Autodesk Fusion 360 part; units mm, degrees
sketch "Skizze1" plane through (0, 0, 0) normal (0, 1, 0) x (1, 0, 0)
  line L0 (7, -7) -> (-7, -7)
  line L1 (-7, -7) -> (-7, 7)
  line L2 (-7, 7) -> (7, 7)
  line L3 (7, 7) -> (7, -7)
  line L4 (7, -7) -> (-7, 7) construction
  line L5 (-7, -7) -> (7, 7) construction
  line L6 (6, 1.65) -> (7, 1.65)
  line L7 (7, 1.65) -> (7, -1.65)
  line L8 (7, -1.65) -> (6, -1.65)
  line L9 (6, -1.65) -> (6, 1.65)
  line L10 (0, 0) -> (-0.0828, 0.0828)
  line L11 (0, 0) -> (0, 4.3114) construction
  line L12 (-7, -1.65) -> (-6, -1.65)
  line L13 (-6, -1.65) -> (-6, 1.65)
  line L14 (-7, 1.65) -> (-7, -1.65)
  line L15 (-6, 1.65) -> (-7, 1.65)
  line L16 (8, -8) -> (-8, -8) construction
  line L17 (-8, -8) -> (-8, 8) construction
  line L18 (-8, 8) -> (8, 8) construction
  line L19 (8, 8) -> (8, -8) construction
  line L20 (8, -8) -> (-8, 8) construction
  line L21 (-8, -8) -> (8, 8) construction
  line L22 (9, -9) -> (-9, -9)
  line L23 (-9, -9) -> (-9, 9)
  line L24 (-9, 9) -> (9, 9)
  line L25 (9, 9) -> (9, -9)
  line L26 (9, -9) -> (-9, 9) construction
  line L27 (-9, -9) -> (9, 9) construction
  line L28 (7, 7) -> (9, 7) construction
  line L29 (25, 8) -> (41, 8) construction
  line L30 (42, 9) -> (42, -9)
  line L31 (40, -7) -> (26, -7)
  line L32 (40, -7) -> (26, 7) construction
  line L33 (25, -8) -> (41, 8) construction
  line L34 (24, 9) -> (42, 9)
  line L35 (26, -7) -> (26, 7)
  line L36 (42, -9) -> (24, -9)
  line L37 (40, -1.65) -> (39, -1.65)
  line L38 (39, 1.65) -> (40, 1.65)
  line L39 (33, 0) -> (33, 4.3114) construction
  line L40 (39, -1.65) -> (39, 1.65)
  line L41 (40, 7) -> (40, -7)
  line L42 (33, 0) -> (32.9172, 0.0828)
  line L43 (40, 1.65) -> (40, -1.65)
  line L44 (41, 8) -> (41, -8) construction
  line L45 (25, -8) -> (25, 8) construction
  line L46 (40, 7) -> (42, 7) construction
  line L47 (27, -1.65) -> (27, 1.65)
  line L48 (41, -8) -> (25, 8) construction
  line L49 (41, -8) -> (25, -8) construction
  line L50 (26, -7) -> (40, 7) construction
  line L51 (26, 7) -> (40, 7)
  line L52 (42, -9) -> (24, 9) construction
  line L53 (26, 1.65) -> (26, -1.65)
  line L54 (26, -1.65) -> (27, -1.65)
  line L55 (24, -9) -> (24, 9)
  line L56 (27, 1.65) -> (26, 1.65)
  line L57 (24, -9) -> (42, 9) construction
  line L58 (33, -34) -> (33, -29.6886) construction
  line L59 (41, -42) -> (25, -26) construction
  line L60 (40, -41) -> (26, -27) construction
  line L61 (25, -42) -> (41, -26) construction
  line L62 (39, -35.65) -> (39, -32.35)
  line L63 (24, -43) -> (42, -25) construction
  line L64 (24, -25) -> (42, -25)
  line L65 (24, -43) -> (24, -25)
  line L66 (26, -41) -> (40, -27) construction
  line L67 (40, -27) -> (42, -27) construction
  line L68 (41, -26) -> (41, -42) construction
  line L69 (26, -32.35) -> (26, -35.65)
  line L70 (25, -42) -> (25, -26) construction
  line L71 (41, -42) -> (25, -42) construction
  line L72 (27, -35.65) -> (27, -32.35)
  line L73 (40, -35.65) -> (39, -35.65)
  line L74 (42, -43) -> (24, -43)
  line L75 (40, -41) -> (26, -41)
  line L76 (26, -41) -> (26, -27)
  line L77 (26, -35.65) -> (27, -35.65)
  line L78 (42, -43) -> (24, -25) construction
  line L79 (27, -32.35) -> (26, -32.35)
  line L80 (25, -26) -> (41, -26) construction
  line L81 (42, -25) -> (42, -43)
  line L82 (9, -43) -> (-9, -25) construction
  line L83 (8, -42) -> (-8, -42) construction
  line L84 (39, -32.35) -> (40, -32.35)
  line L85 (40, -32.35) -> (40, -35.65)
  line L86 (0, -34) -> (-0.0828, -33.9172)
  line L87 (-7, -35.65) -> (-6, -35.65)
  line L88 (8, -26) -> (8, -42) construction
  line L89 (6, -32.35) -> (7, -32.35)
  line L90 (0, -34) -> (0, -29.6886) construction
  line L91 (-9, -43) -> (9, -25) construction
  line L92 (7, -32.35) -> (7, -35.65)
  line L93 (7, -35.65) -> (6, -35.65)
  line L94 (7, -27) -> (7, -41)
  line L95 (6, -35.65) -> (6, -32.35)
  line L96 (-6, -32.35) -> (-7, -32.35)
  line L97 (-9, -43) -> (-9, -25)
  line L98 (9, -25) -> (9, -43)
  line L99 (-8, -26) -> (8, -26) construction
  line L100 (-8, -42) -> (-8, -26) construction
  line L101 (7, -41) -> (-7, -27) construction
  line L102 (-9, -25) -> (9, -25)
  line L103 (7, -27) -> (9, -27) construction
  line L104 (-7, -41) -> (-7, -27)
  line L105 (8, -42) -> (-8, -26) construction
  line L106 (-7, -32.35) -> (-7, -35.65)
  line L107 (-7, -27) -> (7, -27)
  line L108 (-6, -35.65) -> (-6, -32.35)
  line L109 (7, -41) -> (-7, -41)
  line L110 (-8, -42) -> (8, -26) construction
  line L111 (-7, -41) -> (7, -27) construction
  line L112 (9, -43) -> (-9, -43)
  line L113 (33, -34) -> (32.9172, -33.9172)
  line L114 (40, -27) -> (40, -41)
  line L115 (26, -27) -> (40, -27)
  line L116 (68, -34) -> (67.9172, -33.9172)
  line L117 (60, -42) -> (60, -26) construction
  line L118 (61, -41) -> (61, -27)
  line L119 (61, -35.65) -> (62, -35.65)
  line L120 (62, -32.35) -> (61, -32.35)
  line L121 (61, -32.35) -> (61, -35.65)
  line L122 (68, -34) -> (68, -29.6886) construction
  line L123 (61, -7) -> (61, 7)
  line L124 (62, -35.65) -> (62, -32.35)
  line L125 (59, -43) -> (59, -25)
  line L126 (68, 0) -> (68, 4.3114) construction
  line L127 (68, 0) -> (67.9172, 0.0828)
  line L128 (61, -7) -> (75, 7) construction
  line L129 (59, -9) -> (59, 9)
  line L130 (62, -1.65) -> (62, 1.65)
  line L131 (61, -1.65) -> (62, -1.65)
  line L132 (75, -7) -> (61, 7) construction
  line L133 (62, 1.65) -> (61, 1.65)
  line L134 (61, 1.65) -> (61, -1.65)
  line L135 (60, -8) -> (60, 8) construction
  line L136 (77, -25) -> (77, -43)
  line L137 (74, -32.35) -> (75, -32.35)
  line L138 (77, -9) -> (59, 9) construction
  line L139 (75, -32.35) -> (75, -35.65)
  line L140 (75, -35.65) -> (74, -35.65)
  line L141 (75, -27) -> (75, -41)
  line L142 (76, -26) -> (76, -42) construction
  line L143 (76, -8) -> (60, 8) construction
  line L144 (74, -35.65) -> (74, -32.35)
  line L145 (75, -27) -> (77, -27) construction
  line L146 (59, -9) -> (77, 9) construction
  line L147 (74, 1.65) -> (75, 1.65)
  line L148 (60, -8) -> (76, 8) construction
  line L149 (76, -8) -> (60, -8) construction
  line L150 (60, -26) -> (76, -26) construction
  line L151 (75, -41) -> (61, -41)
  line L152 (61, -27) -> (75, -27)
  line L153 (60, -42) -> (76, -26) construction
  line L154 (76, -42) -> (60, -26) construction
  line L155 (77, -9) -> (59, -9)
  line L156 (75, 7) -> (77, 7) construction
  line L157 (59, 9) -> (77, 9)
  line L158 (76, 8) -> (76, -8) construction
  line L159 (59, -25) -> (77, -25)
  line L160 (75, 1.65) -> (75, -1.65)
  line L161 (61, -41) -> (75, -27) construction
  line L162 (77, 9) -> (77, -9)
  line L163 (76, -42) -> (60, -42) construction
  line L164 (60, 8) -> (76, 8) construction
  line L165 (77, -43) -> (59, -25) construction
  line L166 (75, -1.65) -> (74, -1.65)
  line L167 (75, -41) -> (61, -27) construction
  line L168 (59, -43) -> (77, -25) construction
  line L169 (77, -43) -> (59, -43)
  line L170 (61, 7) -> (75, 7)
  line L171 (75, 7) -> (75, -7)
  line L172 (74, -1.65) -> (74, 1.65)
  line L173 (75, -7) -> (61, -7)
  line L174 (-9, -9) -> (77, -9)
  line L175 (77, -9) -> (77, -25)
  line L176 (77, -25) -> (-9, -25)
  line L177 (-9, -25) -> (-9, -9)
  line L178 (42, 9) -> (59, 9)
  line L179 (59, 9) -> (59, -9)
  line L180 (59, -9) -> (42, -9)
  line L181 (42, -9) -> (42, 9)
  line L182 (9, 9) -> (24, 9)
  line L183 (24, 9) -> (24, -9)
  line L184 (24, -9) -> (9, -9)
  line L185 (9, -9) -> (9, 9)
  line L186 (9, -25) -> (24, -25)
  line L187 (24, -25) -> (24, -43)
  line L188 (24, -43) -> (9, -43)
  line L189 (9, -43) -> (9, -25)
  line L190 (42, -25) -> (59, -25)
  line L191 (59, -25) -> (59, -43)
  line L192 (59, -43) -> (42, -43)
  line L193 (42, -43) -> (42, -25)
  line L194 (-9, -43) -> (77, -43)
  line L195 (77, -43) -> (77, -53)
  line L196 (77, -53) -> (-9, -53)
  line L197 (-9, -53) -> (-9, -43)
  line L198 (77, 9) -> (-9, 9)
  line L199 (-9, 9) -> (-9, 19)
  line L200 (-9, 19) -> (77, 19)
  line L201 (77, 19) -> (77, 9)
  line L202 (77, 19) -> (77, 19)
  line L203 (77, 19) -> (77, -53)
  line L204 (77, -53) -> (77, -53)
  line L205 (77, -53) -> (77, 19)
  line L206 (77, -53) -> (87.1689, -53)
  line L207 (87.1689, -53) -> (87.1689, 19)
  line L208 (87.1689, 19) -> (77, 19)
  line L209 (77, 19) -> (77, -53)
  line L210 (-9, -53) -> (-19.4967, -53)
  line L211 (-19.4967, -53) -> (-19.4967, 19)
  line L212 (-19.4967, 19) -> (-9, 19)
  line L213 (-9, 19) -> (-9, -53)
  point P0 (33, 0)
  point P1 (33, 0)
  point P2 (33, 0)
  point P3 (0, -34)
  point P4 (0, -34)
  point P5 (0, -34)
  point P6 (33, -34)
  point P7 (33, -34)
  point P8 (33, -34)
  point P9 (68, 0)
  point P10 (68, 0)
  point P11 (68, 0)
  point P12 (68, -34)
  point P13 (68, -34)
  point P14 (68, -34)
  dimension "d1" = 14
  dimension "d2" = 14
  dimension "d6" = 1
  dimension "d7" = 3.3
  dimension "d8" = 16
  dimension "d9" = 16
  dimension "d10" = 18
  dimension "d11" = 18
  dimension "d13" = 2
  dimension "d19" = 14
  dimension "d20" = 14
  dimension "d21" = 1
  dimension "d22" = 3.3
  dimension "d23" = 16
  dimension "d24" = 16
  dimension "d25" = 18
  dimension "d26" = 18
  dimension "d27" = 2
  dimension "d28" = 14
  dimension "d29" = 14
  dimension "d30" = 1
  dimension "d31" = 3.3
  dimension "d32" = 16
  dimension "d33" = 16
  dimension "d34" = 18
  dimension "d35" = 18
  dimension "d36" = 2
  dimension "d37" = 14
  dimension "d38" = 14
  dimension "d39" = 1
  dimension "d40" = 3.3
  dimension "d41" = 16
  dimension "d42" = 16
  dimension "d43" = 18
  dimension "d44" = 18
  dimension "d45" = 2
  dimension "d46" = 14
  dimension "d47" = 14
  dimension "d48" = 1
  dimension "d49" = 3.3
  dimension "d50" = 16
  dimension "d51" = 16
  dimension "d52" = 18
  dimension "d53" = 18
  dimension "d54" = 2
  dimension "d55" = 14
  dimension "d56" = 14
  dimension "d57" = 1
  dimension "d58" = 3.3
  dimension "d59" = 16
  dimension "d60" = 16
  dimension "d61" = 18
  dimension "d62" = 18
  dimension "d63" = 2
extrude "Extrusion2" add sketch "Skizze1" along normal blind 1.5 contours L3 L6 L7 L8 L9 | L1 L12 L13 L14 L15 | L22 L36 L64 L102 L155 L159 L174 L175 L176 L177 L180 L184 L186 L190 L203 L205 L209 L213 | L22 L23 L24 L25 L174 L185 L198 L213 | L25 L55 L174 L182 L183 L184 L185 L198 | L23 L97 L177 L197 L199 L210 L211 L212 L213 | L24 L34 L157 L178 L182 L198 L199 L200 L201 L203 L205 L209 L213 | L30 L34 L36 L55 L174 L181 L183 L198 | L97 L98 L102 L112 L176 L189 L194 L213 | L30 L129 L174 L178 L179 L180 L181 L198 | L74 L112 L169 L188 L192 L194 L195 L196 L197 L203 L205 L209 L213 | L65 L98 L176 L186 L187 L188 L189 L194 | L129 L155 L157 L162 L174 L179 L198 L203 L205 L209 | L136 L162 L175 L195 L201 L203 L205 L206 L207 L208 L209 | L64 L65 L74 L81 L176 L187 L193 L194 | L81 L125 L176 L190 L191 L192 L193 L194 | L125 L136 L159 L169 L176 L191 L194 L203 L205 L209 | L37 L38 L40 L41 L43 | L35 L47 L53 L54 L56 | L62 L73 L84 L85 L114 | L69 L72 L76 L77 L79 | L87 L96 L104 L106 L108 | L89 L92 L93 L94 L95 | L118 L119 L120 L121 L124 | L137 L139 L140 L141 L144 | L123 L130 L131 L133 L134 | L147 L160 L166 L171 L172
extrude "Extrusion1" [suppressed]
chamfer "Fase1" [suppressed]
equation "d11 = d10"
equation "d26 = d10"
equation "d35 = d10"
equation "d44 = d10"
equation "d53 = d10"
equation "d62 = d10"
Design review of the part built by this model. Coordinates are the model's own, in mm. Coordinates: 2 decimals unless noted, no trailing zeros. Loops run counter-clockwise (first coordinate to the right, second up) from the corner with the lowest first, then second, coordinate; pieces in that order, holes last. Notation, with made-up numbers: (-2.5, -20.75) -> (36.5, -20.75) arc R21 ccw to (36.5, 12.25) -> close; hole circle Ø2 at (72.5, -5.5). An arc over 180 degrees is marked (long way). Use a Markdown table: item, result. Add a question column.
Item 1: We need section A-A, the plane x = 0. Write out the cut boundary in (y, z), and give its area (3 significant figures).
Item 2: Wall thickness on L1, parallel to Z at x = 30, y = 1.15; L2, parallel to X at y = 0.85, z = -1; L3, parallel to X at y = 1, z = 29: over which ranges is each line inside the solid? List them lowest first. Write a range as from..to.
Item 3: We need section B-B, the plane y = 0.25. Count the separate pieces of the cut face and the enclosed holes in it, and give its area (3 significant figures).
Numbers:
| question | item | result |
|---|---|---|
| 1 | outline | (0, -19) -> (1.5, -19) -> (1.5, -7) -> (0, -7) -> close; (0, 7) -> (1.5, 7) -> (1.5, 27) -> (0, 27) -> close; (0, 41) -> (1.5, 41) -> (1.5, 53) -> (0, 53) -> close |
| 1 | area | 66.0 mm^2 |
| 2 | L1 | z = -19..-7, 7..27, 41..53 |
| 2 | L2 | x = -19.5..-6, 6..27, 39..62, 74..87.17 |
| 2 | L3 | x = -19.5..-7, 7..26, 40..61, 75..87.17 |
| 3 | separate pieces | 1 |
| 3 | enclosed holes | 6 |
| 3 | area | 6,540 mm^2 |
